Work out the finished part from the listing and answer in its coordinate system (mm). Coordinates: 2 decimals unless noted, no trailing zeros. Write each loop counter-clockwise with the first axis right and the second up, starting at its lowest first coordinate (ties: lowest second). Pieces come first, ordered by that corner, then holes. Notation, with made-up numbers: (-37.5, 27.5) -> (18.5, 27.5) arc R24 cw to (18.5, 41.5) -> close; hole circle Ø5 at (78, 40.5). An arc over 180 degrees is marked (long way). Write each question's results on one line, items separated by ' | '. Start each with the question number.
from build123d import *

# Parameters (mm, degrees)
SKETCH1_W             = 200
SKETCH1_H             = 20
BOSS_EXTRUDE1_DEPTH   = 6.35
M3X0_5_TAPPED_HOLE1_D = 2.5
M6_CLEARANCE_HOLE1_D  = 6.6


with BuildPart() as part:
    # Sketch1 → Boss-Extrude1 (new body)
    with BuildSketch(Plane(origin=(0, 0, 0), x_dir=(1, 0, 0), z_dir=(0, 1, 0))):
        with Locations((100, 10)):
            Rectangle(SKETCH1_W, SKETCH1_H)
    extrude(amount=BOSS_EXTRUDE1_DEPTH)

    # M3x0.5 Tapped Hole1 (through all)
    with Locations(Plane(origin=(0, 6.35, 0), x_dir=(1, 0, 0), z_dir=(0, 1, 0))):
        with Locations((30, 10), (170, 10), (90, 10)):
            Hole(M3X0_5_TAPPED_HOLE1_D / 2)

    # M6 Clearance Hole1 (through all)
    with Locations(Plane(origin=(0, 6.35, 0), x_dir=(1, 0, 0), z_dir=(0, 1, 0))):
        with Locations((10, 10), (190, 10)):
            Hole(M6_CLEARANCE_HOLE1_D / 2)


solid = part.part
1. Determine the mould class of faces 1 (the face through (12.619, 3.131, -7.992)), 2 (the face through (99, 0, -10)), 3 (the face through (99, 3, -20)) for opening direction Z: pulls with the +Z half, pulls with the -Z half, needs draft (parallel to the pull), parting line crosses it, or undercut.
2. Find section A-A on x = 190. Give the vertices of the cut face in (y, z).
3. Find the intervals of material crossed by L1, parallel to X at y = 2, z = -10; L2, parallel to Z at x = 170, y = 3.5; L3, parallel to X at y = 5, z = -11.5, in increasing order.
4. Find section B-B on y = 3.5. Give the vertices of the cut face in (x, z).
Ans:
1) face 1: undercut | face 2: needs draft | face 3: pulls with the -Z half
2) outline: (0, -20) -> (6.35, -20) -> (6.35, -13.3) -> (0, -13.3) -> close; (0, -6.7) -> (6.35, -6.7) -> (6.35, 0) -> (0, 0) -> close
3) L1: x = 0 to 6.7, 13.3 to 28.75, 31.25 to 88.75, 91.25 to 168.75, 171.25 to 186.7, 193.3 to 200 | L2: z = -20 to -11.25, -8.75 to 0 | L3: x = 0 to 7.06, 12.94 to 187.06, 192.94 to 200
4) outline: (0, -20) -> (200, -20) -> (200, 0) -> (0, 0) -> close; hole circle Ø6.6 at (10, -10); hole circle Ø2.5 at (30, -10); hole circle Ø2.5 at (90, -10); hole circle Ø2.5 at (170, -10); hole circle Ø6.6 at (190, -10)
